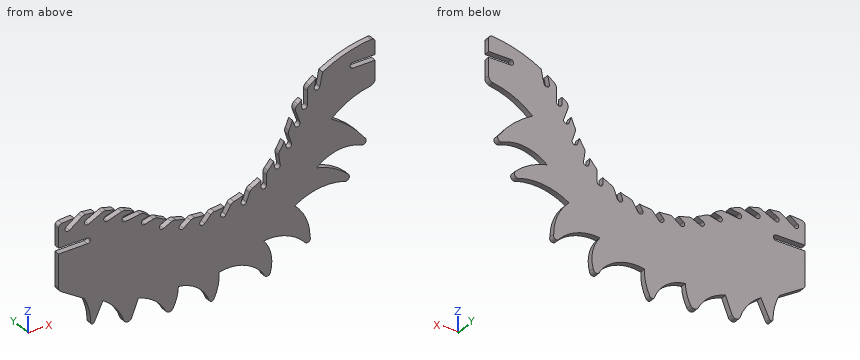
from build123d import *

# Parameters (mm, degrees)
BOSS_EXTRUDE1_DEPTH = 3
FILLET1_R           = 3
FILLET2_R           = 2
FILLET3_R           = 3


with BuildPart() as part:
    # Sketch1 → Boss-Extrude1 (new body)
    with BuildSketch(Plane(origin=(0, 0, 0), x_dir=(1, 0, 0), z_dir=(0, 1, 0))):
        with BuildLine():
            Line((0, 0), (-11.9, 0))
            ThreePointArc((-11.9, 0), (-13.4, -1.5), (-11.9, -3))
            Line((-11.9, -3), (0, -3))
            Line((0, -3), (0, -11.81))
            ThreePointArc((0, -11.81), (-14.472760581, -9.33127549), (-28, -3.62))
            Line((-28, -3.62), (-29.521164874, 3.544255393))
            ThreePointArc((-29.521164874, 3.544255393), (-31.3, 4.7), (-32.455744607, 2.921164874))
            Line((-32.455744607, 2.921164874), (-31.51276538, -1.52))
            Line((-31.51276538, -1.52), (-36.154254994, 1.95))
            Line((-36.154254994, 1.95), (-36.154254994, 10.96))
            ThreePointArc((-36.154254994, 10.96), (-37.654254994, 12.46), (-39.154254994, 10.96))
            Line((-39.154254994, 10.96), (-39.154254994, 7.21))
            Line((-39.154254994, 7.21), (-43.054254994, 10.02))
            Line((-43.054254994, 10.02), (-40.045722247, 18.391072762))
            ThreePointArc((-40.045722247, 18.391072762), (-40.95, 20.31), (-42.868927238, 19.405722247))
            Line((-42.868927238, 19.405722247), (-44.082149392, 16.03))
            ThreePointArc((-44.082149392, 16.03), (-45.222319739, 18.964571548), (-46.49969517, 21.842072304))
            Line((-46.49969517, 21.842072304), (-44.579329128, 27.922952603))
            ThreePointArc((-44.579329128, 27.922952603), (-45.557981292, 29.805036539), (-47.440065228, 28.826384375))
            Line((-47.440065228, 28.826384375), (-48.445885934, 25.641431517))
            ThreePointArc((-48.445885934, 25.641431517), (-49.939100175, 28.203829515), (-51.544744053, 30.697317034))
            Line((-51.544744053, 30.697317034), (-50.573219985, 36.999780991))
            ThreePointArc((-50.573219985, 36.999780991), (-51.827184167, 38.710796429), (-53.538199605, 37.456832246))
            Line((-53.538199605, 37.456832246), (-54.047050003, 34.155821602))
            ThreePointArc((-54.047050003, 34.155821602), (-55.913215675, 36.460815735), (-57.88, 38.680575111))
            Line((-57.88, 38.680575111), (-57.88, 45.057479607))
            ThreePointArc((-57.88, 45.057479607), (-59.38, 46.557479607), (-60.88, 45.057479607))
            Line((-60.88, 45.057479607), (-60.88, 41.717479607))
            ThreePointArc((-60.88, 41.717479607), (-63.667068497, 43.264182629), (-66.54, 44.644872898))
            Line((-66.54, 44.644872898), (-68.597785529, 50.298592173))
            ThreePointArc((-68.597785529, 50.298592173), (-70.520354675, 51.195100889), (-71.416863391, 49.272531743))
            Line((-71.416863391, 49.272531743), (-70.278571651, 46.145100889))
            ThreePointArc((-70.278571651, 46.145100889), (-73.347472166, 47.144625873), (-76.47028294, 47.960256574))
            Line((-76.47028294, 47.960256574), (-79.573687895, 53.114662515))
            ThreePointArc((-79.573687895, 53.114662515), (-81.632457597, 53.626001263), (-82.143796345, 51.567231561))
            Line((-82.143796345, 51.567231561), (-80.427106156, 48.716002593))
            ThreePointArc((-80.427106156, 48.716002593), (-83.630695873, 49.108702849), (-86.851944729, 49.310584926))
            Line((-86.851944729, 49.310584926), (-90.88586279, 53.774498903))
            ThreePointArc((-90.88586279, 53.774498903), (-93.004472595, 53.881701959), (-93.111675651, 51.763092154))
            Line((-93.111675651, 51.763092154), (-90.880259623, 49.293818102))
            ThreePointArc((-90.880259623, 49.293818102), (-94.099716335, 49.065128247), (-97.299926084, 48.645773825))
            Line((-97.299926084, 48.645773825), (-102.114737888, 52.253627786))
            ThreePointArc((-102.114737888, 52.253627786), (-104.214607854, 51.952718952), (-103.913699021, 49.852848986))
            Line((-103.913699021, 49.852848986), (-101.250321117, 47.857116046))
            ThreePointArc((-101.250321117, 47.857116046), (-104.366234103, 47.015518263), (-107.426707901, 45.990481337))
            Line((-107.426707901, 45.990481337), (-112.84383048, 48.608458779))
            ThreePointArc((-112.84383048, 48.608458779), (-114.847075732, 47.910598865), (-114.149215819, 45.907353613))
            Line((-114.149215819, 45.907353613), (-111.152661609, 44.459184182))
            ThreePointArc((-111.152661609, 44.459184182), (-114.049460622, 43.035893612), (-116.856684479, 41.443193143))
            Line((-116.856684479, 41.443193143), (-122.675194955, 42.974192412))
            ThreePointArc((-122.675194955, 42.974192412), (-124.507514461, 41.905265274), (-123.438587323, 40.072945768))
            Line((-123.438587323, 40.072945768), (-120.22, 39.226052931))
            ThreePointArc((-120.22, 39.226052931), (-122.130810504, 37.91089066), (-124.085404111, 36.661725973))
            Line((-124.085404111, 36.661725973), (-133.201211912, 37.826139832))
            ThreePointArc((-133.201211912, 37.826139832), (-134.879181598, 36.528288634), (-133.5813304, 34.850318948))
            Line((-133.5813304, 34.850318948), (-128.447772492, 34.194580466))
            ThreePointArc((-128.447772492, 34.194580466), (-131.166271961, 32.86279471), (-133.941398342, 31.653428662))
            Line((-133.941398342, 31.653428662), (-142.747666571, 34.280870646))
            ThreePointArc((-142.747666571, 34.280870646), (-144.613912239, 33.272343449), (-143.605385042, 31.406097782))
            Line((-143.605385042, 31.406097782), (-138.64614403, 29.926456496))
            ThreePointArc((-138.64614403, 29.926456496), (-141.544646969, 29.053202022), (-144.4791725, 28.309930489))
            Line((-144.4791725, 28.309930489), (-152.742718566, 32.330828141))
            ThreePointArc((-152.742718566, 32.330828141), (-154.747823596, 31.638329899), (-154.055325354, 29.633224868))
            Line((-154.055325354, 29.633224868), (-149.401717777, 27.368860438))
            ThreePointArc((-149.401717777, 27.368860438), (-152.403474262, 26.977260292), (-155.41969517, 26.719764481))
            Line((-155.41969517, 26.719764481), (-162.921707309, 32.027647804))
            ThreePointArc((-162.921707309, 32.027647804), (-165.012578204, 31.669515289), (-164.654445689, 29.578644394))
            Line((-164.654445689, 29.578644394), (-160.42969517, 26.589515289))
            ThreePointArc((-160.42969517, 26.589515289), (-164.583860714, 26.762024861), (-168.71969517, 27.188316155))
            Line((-168.71969517, 27.188316155), (-168.71969517, 39.428316155))
            Line((-168.71969517, 39.428316155), (-153.26969517, 39.428316155))
            ThreePointArc((-153.26969517, 39.428316155), (-151.76969517, 40.928316155), (-153.26969517, 42.428316155))
            Line((-153.26969517, 42.428316155), (-168.71969517, 42.428316155))
            Line((-168.71969517, 42.428316155), (-168.71969517, 61.718316155))
            Line((-168.71969517, 61.718316155), (-154.97969517, 70.548316155))
            ThreePointArc((-154.97969517, 70.548316155), (-152.427356059, 77.262330075), (-151.55969517, 84.392518181))
            ThreePointArc((-151.55969517, 84.392518181), (-150.818108815, 85.328316155), (-149.737615052, 84.820180937))
            ThreePointArc((-149.737615052, 84.820180937), (-147.382689286, 79.982663325), (-145.105861662, 75.107900975))
            ThreePointArc((-145.105861662, 75.107900975), (-138.338315476, 81.303798165), (-133.956265042, 89.365215991))
            ThreePointArc((-133.956265042, 89.365215991), (-131.871910246, 90.88119984), (-129.731541419, 89.445385354))
            Line((-129.731541419, 89.445385354), (-126.235861662, 80.434580466))
            ThreePointArc((-126.235861662, 80.434580466), (-117.683005247, 84.724454595), (-111.681225051, 92.176501788))
            ThreePointArc((-111.681225051, 92.176501788), (-109.702148951, 93.419160866), (-107.687529176, 92.234994088))
            ThreePointArc((-107.687529176, 92.234994088), (-105.674016695, 87.172361666), (-104.865861662, 81.78428548))
            ThreePointArc((-104.865861662, 81.78428548), (-94.760346639, 85.983021815), (-88.401689579, 94.889104066))
            ThreePointArc((-88.401689579, 94.889104066), (-87.233402896, 95.774045948), (-85.956947781, 95.053852748))
            ThreePointArc((-85.956947781, 95.053852748), (-83.657021666, 88.648283331), (-83.100317918, 81.865137997))
            ThreePointArc((-83.100317918, 81.865137997), (-69.828381219, 82.918079825), (-59.38, 91.169402151))
            ThreePointArc((-59.38, 91.169402151), (-57.567745971, 92.98165618), (-55.755491942, 91.169402151))
            ThreePointArc((-55.755491942, 91.169402151), (-55.490451605, 82.06533391), (-59.38, 73.829696824))
            ThreePointArc((-59.38, 73.829696824), (-47.491282563, 75.241319694), (-37.654254994, 82.06533391))
            ThreePointArc((-37.654254994, 82.06533391), (-35.386857444, 82.701978015), (-34.750213339, 80.434580466))
            ThreePointArc((-34.750213339, 80.434580466), (-36.797944646, 70.007982254), (-42.868927238, 61.287298558))
            ThreePointArc((-42.868927238, 61.287298558), (-30.212205095, 56.590662372), (-16.746463394, 57.5523314))
            ThreePointArc((-16.746463394, 57.5523314), (-14.115302595, 57.148635399), (-14.518998596, 54.5174746))
            ThreePointArc((-14.518998596, 54.5174746), (-22.213696249, 48.822896746), (-31.178351733, 45.465585178))
            ThreePointArc((-31.178351733, 45.465585178), (-19.97556246, 40.118304816), (-7.665463567, 41.717479607))
            ThreePointArc((-7.665463567, 41.717479607), (-5.128000509, 41.21803817), (-5.627441946, 38.680575111))
            ThreePointArc((-5.627441946, 38.680575111), (-13.63807278, 29.672013228), (-23.42, 22.626568355))
            ThreePointArc((-23.42, 22.626568355), (-12.55613394, 15.556844164), (0, 12.34))
            Line((0, 12.34), (0, 0))
        make_face()
    extrude(amount=BOSS_EXTRUDE1_DEPTH)

    # Fillet1
    fillet1_edges = [part.edges().sort_by_distance(p)[0] for p in [
        (0, 1.5, -12.34),
    ]]
    fillet(fillet1_edges, radius=FILLET1_R)

    # Fillet2
    fillet2_edges = [part.edges().sort_by_distance(p)[0] for p in [
        (0, 1.5, 11.81),
        (-168.71969517, 1.5, -27.188316155),
    ]]
    fillet(fillet2_edges, radius=FILLET2_R)

    # Fillet3
    fillet3_edges = [part.edges().sort_by_distance(p)[0] for p in [
        (-36.154254994, 1.5, -1.95),
        (-43.054254994, 1.5, -10.02),
        (-46.49969517, 1.5, -21.842072304),
        (-51.544744053, 1.5, -30.697317034),
        (-57.88, 1.5, -38.680575111),
        (-66.54, 1.5, -44.644872898),
        (-76.47028294, 1.5, -47.960256574),
        (-86.851944729, 1.5, -49.310584926),
        (-97.299926084, 1.5, -48.645773825),
        (-107.426707901, 1.5, -45.990481337),
        (-116.856684479, 1.5, -41.443193143),
        (-124.085404111, 1.5, -36.661725973),
        (-133.941398342, 1.5, -31.653428662),
        (-144.4791725, 1.5, -28.309930489),
        (-155.41969517, 1.5, -26.719764481),
        (-168.71969517, 1.5, -61.718316155),
    ]]
    fillet(fillet3_edges, radius=FILLET3_R)


solid = part.part
Check sheet for the modelled part. Datum: model origin and axes. Units: mm. Round coordinates to 2 decimals unless told otherwise and drop trailing zeros. Loops run counter-clockwise (first coordinate to the right, second up) from the corner with the lowest first, then second, coordinate; pieces in that order, holes last.
1. Sectioned sample at A-A on z = -68. Record the boundary of the cut face in (x, y), and give its area (3 significant figures).
2. Scan lines: probe 1 along Z at (x, y) = (-16.5, 1.3); probe 2 along Z at (x, y) = (-21, 0.4); probe 3 along X at (y, z) = (0.8, -49.5). Record each from-to range of solid material in increasing order.
3. Gauge pin test, flat ends, axial feed: pin 1 Ø0.9 at (x, y) = (-8, 1.5) entering from +Z (3 decimals); pin 2 Ø0.9 at (y, z) = (1.5, -7.5) entering from -X; pin 3 Ø5 at (x, z) = (-50, -22) entering from +Y; pin 4 Ø1.5 at (x, y) = (-162.5, 1) entering from -Z. Record the tip position at first contact, or that the pin passes through.
Recorded:
1. outline: (-158.95, 0) - (-37.75, 0) - (-37.75, 3) - (-158.95, 3) - close
1. area: 364 mm2
2. probe 1: z = -57.71 to -52.72, -39.85 to -27.26, -17.56 to 8.7
2. probe 2: z = -56.62 to -49.51, -40.31 to -24.08, -20.59 to 7.03
2. probe 3: x = -168.72 to -103.44, -98.44 to -91.07, -86.66 to -80.9, -77.4 to -71.48, -68.31 to -21.02
3. pin 1: stops at z = 10.945
3. pin 2: stops at x = -40.18
3. pin 3: passes through
3. pin 4: stops at z = -66.2
